Drawing for the job (mm, zero at the part's lowest x, y, z). A direction names the side the tool comes from. Coordinates: 2 decimals unless noted, no trailing zeros. Order: outer loops, then holes, each group sorted by start corner. A loop starts at its lowest first (then second) coordinate and runs counter-clockwise, first axis right, second up.
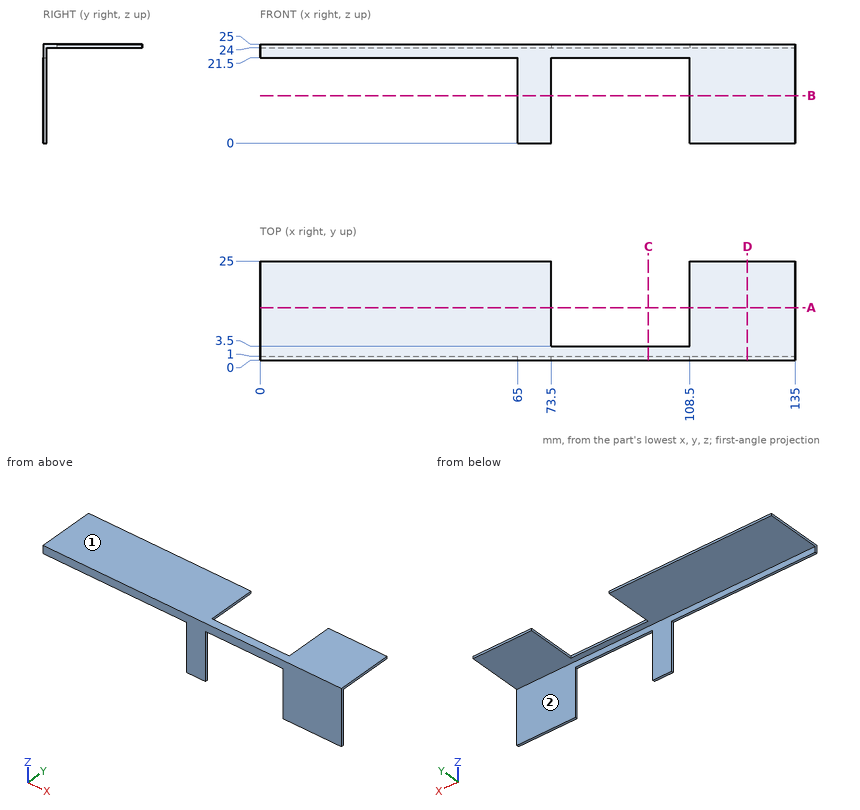
1) Drill centre line: probe 1 along Z at (x, y) = (116, 14.5). Where is it in solid material? Low to high.
2) Slice it at C-C (x = 98). List the corners of the cut face in (y, z).
3) Slice it at A-A (y = 13.25). List the corners of the cut face in (x, z), plus the area to 3 significant figures.
4) Which spindle directions (+Z, -Z, +X, -X, +Y, -Y) get a long thin tool onto all of the face, cutting with end or side? Do the marked faces 1 and 2. Say none if no direction does.
5) Slice it at D-D (x = 123). List the corners of the cut face in (y, z).
6) Pin check, flat tips, straight feed: P1, Ø6, axis at x = 16.5, y = 14, coming from the -Z side; P2, Ø0.8, axis at y = 0.5, z = 14, coming from the -X side; P3, Ø8, axis at y = 20, z = 19.5, coming from the -X side; P4, Ø10, axis at x = 121.5, z = 18.5, coming from the -Y side. Stop position of each tip, or through.
7) Slice it at B-B (z = 12). List the corners of the cut face in (x, y), plus the area to 3 significant figures.
Worked out:
1. probe 1: z = 24 to 25
2. outline: (0, 21.5) - (1, 21.5) - (1, 24) - (3.5, 24) - (3.5, 25) - (0, 25) - close
3. outline: (0, 24) - (73.5, 24) - (73.5, 25) - (0, 25) - close; (108.5, 24) - (135, 24) - (135, 25) - (108.5, 25) - close
3. area: 100 mm2
4. face 1: +Z, +X, -X, +Y, -Y
4. face 2: -Z, +X, -X, +Y
5. outline: (0, 0) - (1, 0) - (1, 24) - (25, 24) - (25, 25) - (0, 25) - close
6. P1: stops at z = 24
6. P2: stops at x = 65
6. P3: passes through
6. P4: stops at y = 0
7. outline: (65, 0) - (73.5, 0) - (73.5, 1) - (65, 1) - close; (108.5, 0) - (135, 0) - (135, 1) - (108.5, 1) - close
7. area: 35.0 mm2
